Part model, mm, in its own coordinate system. A direction names the side the tool comes from. Round coordinates to 2 decimals unless told otherwise and drop trailing zeros. Loops run counter-clockwise (first coordinate to the right, second up) from the corner with the lowest first, then second, coordinate; pieces in that order, holes last. Notation, with made-up numbers: (59, 54) - (92, 54) arc R17 ccw to (92, 84) - close; hole circle Ø7 at (-26, 58). An arc over 180 degrees is marked (long way). Write each question's results on one line, items separated by ' | '. Start each with the question number.
(1) Cut at D-D, the plane x = 19. List the corners of the cut face in (y, z), then the cut area to 3 significant figures.
(2) Drill centre lines: L1, parallel to X at y = 14.5, z = -13; L2, parallel to Y at x = 5, z = -54; L3, parallel to Z at x = 26, y = 14.5. Where is each one in solid material? Low to high.
(3) Cut at B-B, the plane y = 30. List the corners of the cut face in (x, z), then the cut area to 3 significant figures.
(4) Cut at C-C, the plane x = -8.5. List the corners of the cut face in (y, z).
(5) Flat gauge pins, fed straight in: P1, Ø1.5, axis at x = -7, y = 24.5, coming from the -Z side; P2, Ø12, axis at y = 24, z = 9, coming from the -X side; P3, Ø8, axis at y = 9, z = 13, coming from the -X side. Where does each tip first touch, or does it go through?
(6) Cut at A-A, the plane z = 10.5. List the corners of the cut face in (x, y), then the cut area to 3 significant figures.
(7) Tool access for faces 1 (the face through (1.02, 35.14, -79.77)), 2 (the face through (33.79, 35.14, -7.98)), 3 (the face through (-14.234, 35, -43)): list every direction of +Z, -Z, +X, -X, +Y, -Y with a clear straight run to the whole face (end or side of a thin tool).
from build123d import *


with BuildPart() as f2:
    # F2: sweep along a path in F1
    with BuildLine(Plane.YZ) as f2_path:
        Line((0, 0), (69.312386, -68.5388))
    # F0 (on Front) → F2 (sweep)
    with BuildSketch(Plane.XZ):
        Polygon((51.365424, 43.474954), (-44.557959, 43.474954), (-43.939099, 25.527997), (-14.233792, 25.527997), (-14.233792, -45.022104), (16.709233, -45.022104), (16.709233, 26.765719), (51.365424, 26.765719), align=None)
    sweep(path=f2_path.line)


solid = f2.part
A:
1) outline: (0, 26.77) - (69.31, -41.77) - (69.31, -25.06) - (0, 43.47) - close | area: 1,160 mm2
2) L1: -14.23 to 16.71 | L2: 9.08 to 69.31 | L3: 12.43 to 29.14
3) outline: (-44.56, 13.81) - (-43.94, -4.14) - (-14.23, -4.14) - (-14.23, -74.69) - (16.71, -74.69) - (16.71, -2.9) - (51.37, -2.9) - (51.37, 13.81) - close | area: 3,860 mm2
4) outline: (0, -45.02) - (69.31, -113.56) - (69.31, -25.06) - (0, 43.47) - close
5) P1: z = -69.99 | P2: x = -44.48 | P3: x = -44.01
6) outline: (-44.56, 33.35) - (-43.94, 15.2) - (-14.23, 15.2) - (-14.23, 0) - (16.71, 0) - (16.71, 16.45) - (51.37, 16.45) - (51.37, 33.35) - close | area: 2,160 mm2
7) face 1: -Z, +X, -X, -Y | face 2: -Z, +X, -Y | face 3: -Z, -X, -Y
